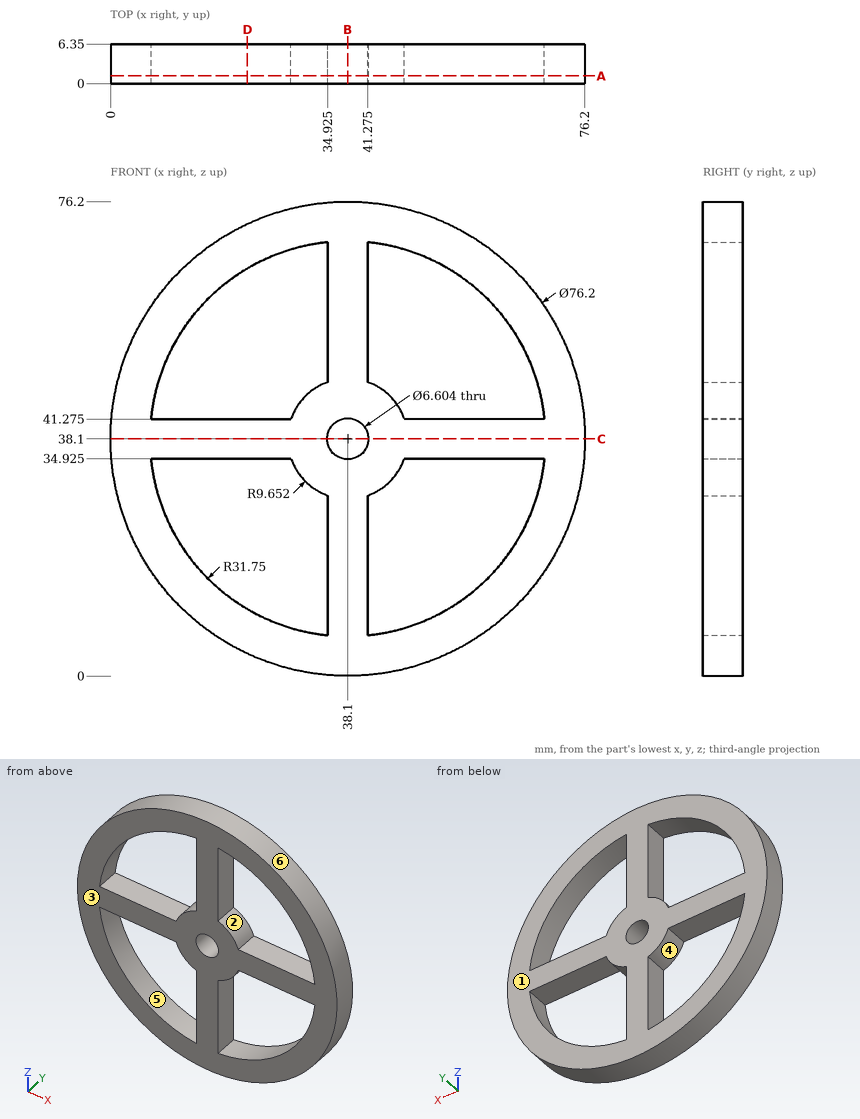
Job drawing, mm, ordinate dimensions from the low corner. One solid piece. A direction names the side the tool comes from. Round coordinates to 2 decimals unless told otherwise and drop trailing zeros. Write each loop counter-clockwise with the first axis right and the second up, starting at its lowest first coordinate (ties: lowest second). Pieces come first, ordered by that corner, then holes. Notation, with made-up numbers: M 20.5,51 L 42.5,51 A19 ccw 42.5,76 Z; hole C 61.5,-32 d7. An arc over 180 degrees is marked long. Return JSON: item names as keys, results as strings. Group by question number.
(1) Saw through at B-B on x = 38.1. Write the cut outline in (y, z), then the cut area to 3 significant figures.
(2) Drill centre lines: probe 1 along Z at (x, y) = (45.5, 3); probe 2 along Z at (x, y) = (19, 0.75) (3 decimals); probe 3 along X at (y, z) = (1.5, 66) (3 decimals). Where is each one in solid material? Low to high.
(3) Saw through at D-D on x = 22. Write the cut outline in (y, z) (3 decimals), then the cut area to 3 significant figures.
(4) Which spindle directions (+Z, -Z, +X, -X, +Y, -Y) get a long thin tool onto all of the face, cutting with end or side? Do the marked faces 1 and 2. Say none if no direction does.
(5) Saw through at A-A on y = 1.25. Write the cut outline in (x, z) (3 decimals).
(6) Two-plate mould, pull along X, no slides. Class the marked faces 3, 4, 5 and 6: +X half, -X half, draft (parallel to the pull), parting line (faces both ways), or undercut.
(7) Pin check, flat tips, straight feed: pin 1 Ø1.9 at (x, y) = (19.5, 4) entering from +Z; pin 2 Ø3 at (x, y) = (17.5, 2.5) entering from -Z; pin 3 Ø10.5 at (x, z) = (38.1, 38.1) entering from -Y; pin 4 Ø1.9 at (x, y) = (53, 3) entering from +Z. Stop position of each tip, or through.
(8) Saw through at C-C on z = 38.1. Write the cut outline in (x, y), then the cut area to 3 significant figures.
Returned:
{
 "1": {"outline": "M 0,0 L 6.35,0 L 6.35,34.8 L 0,34.8 Z; M 0,41.4 L 6.35,41.4 L 6.35,76.2 L 0,76.2 Z", "area": "442 mm²"},
 "2": {"probe 1": "0.73 to 7.22, 31.9 to 44.3, 68.98 to 75.47", "probe 2": "5.133 to 12.738, 34.925 to 41.275, 63.462 to 71.067", "probe 3": "12.154 to 22.946, 34.925 to 41.275, 53.254 to 64.046"},
 "3": {"outline": "M 0,3.569 L 6.35,3.569 L 6.35,10.735 L 0,10.735 Z; M 0,34.925 L 6.35,34.925 L 6.35,41.275 L 0,41.275 Z; M 0,65.465 L 6.35,65.465 L 6.35,72.631 L 0,72.631 Z", "area": "131 mm²"},
 "4": {"face 1": "+Z, -Z, +X, -X, +Y", "face 2": "+Y, -Y"},
 "5": {"outline": "C 38.1,38.1 d76.2; hole M 6.509,34.925 A31.75 ccw 34.925,6.509 L 34.925,28.985 A9.652 cw 28.985,34.925 Z; hole M 6.509,41.275 L 28.985,41.275 A9.652 cw 34.925,47.215 L 34.925,69.691 A31.75 ccw Z; hole C 38.1,38.1 d6.604; hole M 41.275,6.509 A31.75 ccw 69.691,34.925 L 47.215,34.925 A9.652 cw 41.275,28.985 Z; hole M 41.275,47.215 A9.652 cw 47.215,41.275 L 69.691,41.275 A31.75 ccw 41.275,69.691 Z"},
 "6": {"face 3": "draft", "face 4": "undercut", "face 5": "undercut", "face 6": "parting line"},
 "7": {"pin 1": "z = 71.87", "pin 2": "z = 5.13", "pin 3": "y = 0", "pin 4": "z = 73.55"},
 "8": {"outline": "M 0,0 L 34.8,0 L 34.8,6.35 L 0,6.35 Z; M 41.4,0 L 76.2,0 L 76.2,6.35 L 41.4,6.35 Z", "area": "442 mm²"}
}
